Part model, mm, in its own coordinate system. A direction names the side the tool comes from. Give positions to 0.01 mm unless a question says otherwise; leave off trailing zeros. Write each loop counter-clockwise with the first axis right and the second up, starting at its lowest first coordinate (ties: lowest second). Pieces come first, ordered by that corner, then holes. Notation, with made-up numbers: M 12,-22.5 L 25,-22.5 A34 ccw 25,16.5 Z; hole C 19.25,-16.75 d2. An arc over 180 degrees is marked long. Answer as CSV lines item,"result". Start each with the question number.
1) Mould opens along Z. For faces 3 (the cylindrical face through (25.044, 49.601, -774.448)), 4 (the flat face through (25.04, 68.37, -77.72)), 5 (the flat face through (25.044, 152.772, -302.171)) say: pulls with the +Z half, pulls with the -Z half, needs draft (parallel to the pull), parting line crosses it, or undercut.
2) Slice it at A-A, the plane y = 75. Give the cut face in (x, z).
3) Tool access for faces 1 (the flat face through (25.04, 145.41, -301.9)), 2 (the flat face through (0, 143, -391)): list every direction of +Z, -Z, +X, -X, +Y, -Y with a clear straight run to the whole face (end or side of a thin tool).
4) Slice it at C-C, the plane x = 20.5. Give the cut face in (y, z) (3 decimals), plus the area to 3 significant figures.
5) Wall check: line 1 along Y through (x, z) = (18.5, -570); line 2 along Y through (x, z) = (22, -108); line 3 along Z through (x, y) = (22, 35.5). Give the ranges that are in metal, low to high. Write a range as from..to.
6) Pin check, flat tips, straight feed: pin 1 Ø2 at (x, y) = (31, 87.5) entering from -Z; pin 2 Ø12 at (x, y) = (28.5, 74.5) entering from +Z; pin 3 Ø10 at (x, y) = (37.5, 66.5) entering from +Z. Stop position of each tip, or through.
7) Slice it at B-B, the plane z = -72.5. Give the cut face in (x, y).
```python
from build123d import *

# Parameters (mm, degrees)
EXTRUDE_THIN1_DEPTH = 50.8


with BuildPart() as part:
    # Sketch1 → Extrude-Thin1 (new body)
    with BuildSketch(Plane(origin=(0, 0, 0), x_dir=(0, 0, -1), z_dir=(1, 0, 0))):
        with BuildLine():
            Line((737.113874036, 8.511904093), (456.21754645, 5.336904093))
            ThreePointArc((456.21754645, 5.336904093), (455.703672415, 5.334), (455.189798379, 5.336904093))
            Line((455.189798379, 5.336904093), (174.293470793, 8.511904093))
            ThreePointArc((174.293470793, 8.511904093), (160.502158444, 10.818090953), (148.063879552, 17.206205881))
            Line((148.063879552, 17.206205881), (5.379457693, 120.98648949))
            ThreePointArc((5.379457693, 120.98648949), (-2.917750189, 147.368675717), (19.892164793, 163.00744764))
            Line((19.892164793, 163.00744764), (592.464987809, 142.245967303))
            ThreePointArc((592.464987809, 142.245967303), (595.219854288, 141.976498391), (597.921135385, 141.372359959))
            Line((597.921135385, 141.372359959), (749.221113821, 97.654109903))
            ThreePointArc((749.221113821, 97.654109903), (781.652360545, 47.85601599), (737.113874036, 8.511904093))
        make_face()
        with BuildLine():
            Line((737.0306207, 15.877433597), (456.134293115, 12.702433597))
            ThreePointArc((456.134293115, 12.702433597), (455.703672415, 12.7), (455.273051714, 12.702433597))
            Line((455.273051714, 12.702433597), (174.376724129, 15.877433597))
            ThreePointArc((174.376724129, 15.877433597), (162.819758473, 17.809992419), (152.396619736, 23.163161353))
            Line((152.396619736, 23.163161353), (9.712197878, 126.943444962))
            ThreePointArc((9.712197878, 126.943444962), (4.044706155, 144.96406397), (19.625249176, 155.646285228))
            Line((19.625249176, 155.646285228), (592.198072192, 134.884804891))
            ThreePointArc((592.198072192, 134.884804891), (594.055285548, 134.703140457), (595.876373928, 134.29585612))
            Line((595.876373928, 134.29585612), (747.176352364, 90.577606064))
            ThreePointArc((747.176352364, 90.577606064), (774.353374758, 48.847359768), (737.0306207, 15.877433597))
        make_face(mode=Mode.SUBTRACT)
    extrude(amount=EXTRUDE_THIN1_DEPTH)


solid = part.part
```
Found:
1,face 3,"undercut"
1,face 4,"pulls with the +Z half"
1,face 5,"pulls with the -Z half"
2,outline,"M 0,-776.91 L 50.8,-776.91 L 50.8,-768.37 L 0,-768.37 Z; M 0,-81.13 L 50.8,-81.13 L 50.8,-68.6 L 0,-68.6 Z"
3,face 1,"+X, -X"
3,face 2,"+Z, -Z, -X, +Y, -Y"
4,outline,"M 5.337,-456.218 L 8.512,-737.114 A45.466 ccw 97.654,-749.221 L 141.372,-597.921 A22.606 ccw 142.246,-592.465 L 163.007,-19.892 A23.241 ccw 120.986,-5.379 L 17.206,-148.064 A45.466 ccw 8.512,-174.293 L 5.337,-455.19 A45.466 ccw Z; hole M 12.702,-456.134 L 15.877,-737.031 A38.1 ccw 90.578,-747.176 L 134.296,-595.876 A15.24 ccw 134.885,-592.198 L 155.646,-19.625 A15.875 ccw 126.943,-9.712 L 23.163,-152.397 A38.1 ccw 15.877,-174.377 L 12.702,-455.273 A38.1 ccw Z"
4,area,"12,300 mm²"
5,line 1,"6.62..13.99, 135.69..143.06"
5,line 2,"46.35..55.45, 152.44..159.81"
5,line 3,"-778.14..-769.92, -135.44..-122.91"
6,pin 1,"z = -768.37"
6,pin 2,"z = -61.04"
6,pin 3,"z = -73.42"
7,outline,"M 0,72.17 L 50.8,72.17 L 50.8,81.28 L 0,81.28 Z; M 0,153.73 L 50.8,153.73 L 50.8,161.1 L 0,161.1 Z"
